Answer from the drawing. Dimensions are ordinates in mm from the lowest x, y and z of the part. A direction names the side the tool comes from. Round coordinates to 2 decimals unless told otherwise and drop trailing zeros. Loops run counter-clockwise (first coordinate to the right, second up) from the corner with the lowest first, then second, coordinate; pieces in that order, holes last. Notation, with made-up numbers: (-18.75, -12) - (28.25, -12) arc R24 ccw to (28.25, 22) - close; hole circle Ø9 at (84.25, 42). An arc over 180 degrees is marked (long way). Return JSON: item names as keys, results as strings.
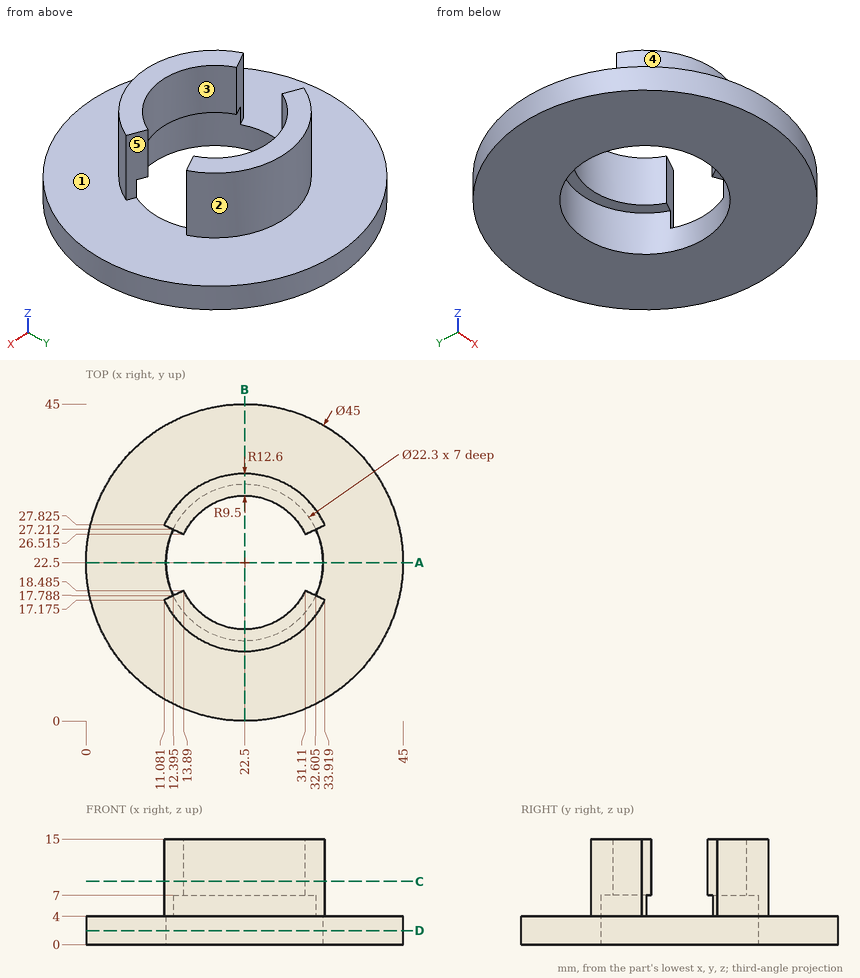
1) A tool of negligible diameter and unlimited length cuts with its end or side. For the marked faces 1, 2, 3, 4 and 5, from which of +Z, -Z, +X, -X, +Y, -Y can it reach the whole face along a straight path? Write none if from no direction.
Verdict:
{"face 1": "+Z", "face 2": "+Z, +Y", "face 3": "+Z, -Z", "face 4": "+Z, -Y", "face 5": "+Z, +X"}
2) Section B-B (x = 22.5) is taken. Give the vertices of the cut face in (y, z), and give its area (3 significant figures).
Verdict:
{"outline": "(0, 0) - (11.35, 0) - (11.35, 7) - (13, 7) - (13, 15) - (9.9, 15) - (9.9, 4) - (0, 4) - close; (32, 7) - (33.65, 7) - (33.65, 0) - (45, 0) - (45, 4) - (35.1, 4) - (35.1, 15) - (32, 15) - close", "area": "149 mm2"}
3) Section A-A (y = 22.5) is taken. Give the vertices of the cut face in (x, z).
Verdict:
{"outline": "(0, 0) - (11.35, 0) - (11.35, 4) - (0, 4) - close; (33.65, 0) - (45, 0) - (45, 4) - (33.65, 4) - close"}
4) Find the intervals of material crossed by L1, parallel to Y at x = 22.5, z = 3.75; L2, parallel to Z at x = 9, y = 34.5; L3, parallel to Z at x = 19, y = 32, in increasing order.
Verdict:
{"L1": "y = 0 to 11.35, 33.65 to 45", "L2": "z = 0 to 4", "L3": "z = 7 to 15"}
5) Section D-D (z = 2) is taken. Give the vertices of the cut face in (x, y).
Verdict:
{"outline": "circle Ø45 at (22.5, 22.5); hole circle Ø22.3 at (22.5, 22.5)"}
6) Section C-C (z = 9) is taken. Give the vertices of the cut face in (x, y) (1 decimal).
Verdict:
{"outline": "(11.1, 17.2) arc R12.6 ccw to (33.9, 17.2) - (31.1, 18.5) arc R9.5 cw to (13.9, 18.5) - close; (11.1, 27.8) - (13.9, 26.5) arc R9.5 cw to (31.1, 26.5) - (33.9, 27.8) arc R12.6 ccw to start"}
7) Flat-ended cylindrical pins translate along their axes: pin 1 (8 mm diameter, centred on y = 12.5, z = 9, fed in from -X); pin 2 (2 mm diameter, centred on x = 18, y = 14.5, fed in from -Z); pin 3 (1 mm diameter, centred on x = 37.5, z = 2, fed in from -Y) (1 decimal); pin 4 (13.5 mm diameter, centred on x = 22.5, y = 22.5, fed in from -Z). Find the tip coordinate at first contact, or state that the pin passes through.
Verdict:
{"pin 1": "stops at x = 11.42", "pin 2": "stops at z = 7", "pin 3": "stops at y = 5.3", "pin 4": "passes through"}
